Verification items for the finished model (mm, model axes). Face numbers are marked on the shaded views. A direction names the side the tool comes from. Round coordinates to 2 decimals unless told otherwise and drop trailing zeros. Write each loop counter-clockwise with the first axis right and the second up, starting at its lowest first coordinate (ties: lowest second). Pieces come first, ordered by that corner, then holes. Notation, with made-up numbers: M 31.5,6.5 L 67.5,6.5 A18 cw 67.5,12.5 Z; hole C 83,69.25 d2. An arc over 180 degrees is marked long. Answer in a Markdown table with one row per item. Add a question column.
1. Material ranges on probe 1 along X at (y, z) = (2.35, 0.5); probe 2 along Z at (x, y) = (40.41, 1.75); probe 3 along Z at (x, y) = (20, 3.8), recorded low to high.
2. Set-up check for the marked faces 1, 2 and 3: record each of +Z, -Z, +X, -X, +Y, -Y from which the full face is reachable in a straight line by a thin tool's end or side.
3. Sectioned sample at C-C on x = 40.41. Record the cut outline in (y, z).
4. Draft check along X on the marked faces 4 and 5. Enter one of: pulls with the +X half, pulls with the -X half, needs draft (parallel to the pull), parting line crosses it, or undercut.
5. Sectioned sample at D-D on x = 16. Record the cut outline in (y, z), plus the area to 3 significant figures.
6. Sectioned sample at A-A on y = 0.45. Record the cut outline in (x, z), plus the area to 3 significant figures.
7. Sectioned sample at B-B on z = 0. Record the cut outline in (x, y), plus the area to 3 significant figures.
8. Go/stop test with flat-tipped pins: pin 1 Ø1.2 at (x, y) = (18, 2) entering from -Z; pin 2 Ø1 at (y, z) = (3, 2) entering from -X; pin 3 Ø2 at (x, y) = (27.5, 1.5) entering from +Z. Record where each tip stops, or that it passes through.
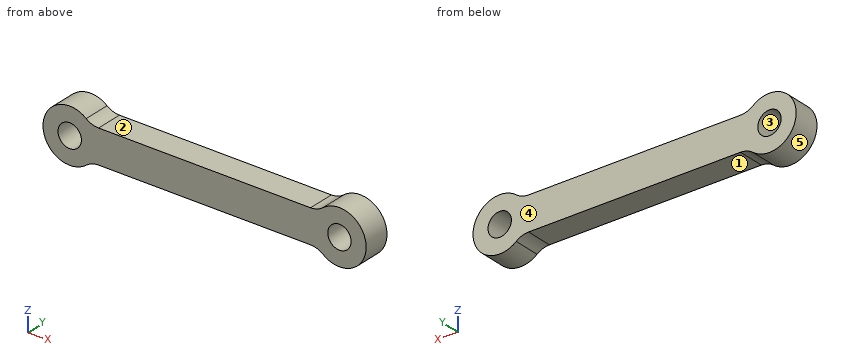
```python
from build123d import *

# Parameters (mm, degrees)
SKETCH1_R           = 1.75
BOSS_EXTRUDE1_DEPTH = 4


with BuildPart() as part:
    # Sketch1 → Boss-Extrude1 (new body)
    with BuildSketch(Plane.XZ):
        with BuildLine():
            Line((36.07987298, 2.5), (4.330127019, 2.5))
            ThreePointArc((4.330127019, 2.5), (3.348146513, 2.665266452), (2.474358297, 3.142857143))
            ThreePointArc((2.474358297, 3.142857143), (-4, 0), (2.474358297, -3.142857143))
            ThreePointArc((2.474358297, -3.142857143), (3.348146513, -2.665266452), (4.330127019, -2.5))
            Line((4.330127019, -2.5), (36.07987298, -2.5))
            ThreePointArc((36.07987298, -2.5), (37.061853486, -2.665266452), (37.935641702, -3.142857143))
            ThreePointArc((37.935641702, -3.142857143), (44.409999999, 0), (37.935641702, 3.142857143))
            ThreePointArc((37.935641702, 3.142857143), (37.061853486, 2.665266452), (36.07987298, 2.5))
        make_face()
        with Locations(Location((40.409999999, 0, 0), (0, 0, 90))):
            Circle(SKETCH1_R, mode=Mode.SUBTRACT)
        with Locations(Location((0, 0, 0), (0, 0, 90))):
            Circle(SKETCH1_R, mode=Mode.SUBTRACT)
    extrude(amount=-BOSS_EXTRUDE1_DEPTH)


solid = part.part
```
Geometry check:
| question | item | result |
|---|---|---|
| 1 | probe 1 | x = -3.97 to -1.68, 1.68 to 38.73, 42.09 to 44.38 |
| 1 | probe 2 | z = -4 to -1.75, 1.75 to 4 |
| 1 | probe 3 | z = -2.5 to 2.5 |
| 2 | face 1 | -Z, +Y, -Y |
| 2 | face 2 | +Z, +Y, -Y |
| 2 | face 3 | +Y, -Y |
| 3 | outline | M 0,-4 L 4,-4 L 4,-1.75 L 0,-1.75 Z; M 0,1.75 L 4,1.75 L 4,4 L 0,4 Z |
| 4 | face 4 | needs draft |
| 4 | face 5 | undercut |
| 5 | outline | M 0,-2.5 L 4,-2.5 L 4,2.5 L 0,2.5 Z |
| 5 | area | 20.0 mm2 |
| 6 | outline | M 2.47,-3.14 A3 cw 4.33,-2.5 L 36.08,-2.5 A3 cw 37.94,-3.14 A4 ccw long 37.94,3.14 A3 cw 36.08,2.5 L 4.33,2.5 A3 cw 2.47,3.14 A4 ccw long Z; hole C 0,0 d3.5; hole C 40.41,0 d3.5 |
| 6 | area | 247 mm2 |
| 7 | outline | M -4,0 L -1.75,0 L -1.75,4 L -4,4 Z; M 1.75,0 L 38.66,0 L 38.66,4 L 1.75,4 Z; M 42.16,0 L 44.41,0 L 44.41,4 L 42.16,4 Z |
| 7 | area | 166 mm2 |
| 8 | pin 1 | stops at z = -2.5 |
| 8 | pin 2 | stops at x = -3.71 |
| 8 | pin 3 | stops at z = 2.5 |
